from build123d import *

# Parameters (mm, degrees)
SKETCH3_W           = 304.8
SKETCH3_H           = 669.93516
SKETCH3_W_2         = 25.4
SKETCH3_H_2         = 3.175
SKETCH3_W_3         = 3.175
SKETCH3_H_3         = 25.4
BOSS_EXTRUDE1_DEPTH = 3.175
SKETCH6_W           = 107.287119944
SKETCH6_H           = 30.1625
SKETCH6_W_2         = 38.1
SKETCH6_H_2         = 114.3
BOSS_EXTRUDE2_DEPTH = 3.175


with BuildPart() as part:
    # Sketch3 → Boss-Extrude1 (new body)
    with BuildSketch(Plane(origin=(0, 0, 0), x_dir=(1, 0, 0), z_dir=(0, 1, 0))):
        with Locations((48.58004, 334.96758)):
            Rectangle(SKETCH3_W, SKETCH3_H)
        with Locations((25.4, 448.21094)):
            Rectangle(SKETCH3_W_2, SKETCH3_H_2, mode=Mode.SUBTRACT)
        with Locations((175.58004, 448.21094)):
            Rectangle(SKETCH3_W_2, SKETCH3_H_2, mode=Mode.SUBTRACT)
        with Locations((100.49002, 448.21094)):
            Rectangle(SKETCH3_W_2, SKETCH3_H_2, mode=Mode.SUBTRACT)
        with Locations((100.49002, 647.71016)):
            Rectangle(SKETCH3_W_3, SKETCH3_H_3, mode=Mode.SUBTRACT)
        with Locations((100.49002, 475.19844)):
            Rectangle(SKETCH3_W_3, SKETCH3_H_3, mode=Mode.SUBTRACT)
        with Locations((100.49002, 561.4543)):
            Rectangle(SKETCH3_W_3, SKETCH3_H_3, mode=Mode.SUBTRACT)
        with Locations((100.49002, 421.22344)):
            Rectangle(SKETCH3_W_3, SKETCH3_H_3, mode=Mode.SUBTRACT)
        with Locations((100.49002, 334.96758)):
            Rectangle(SKETCH3_W_3, SKETCH3_H_3, mode=Mode.SUBTRACT)
        with Locations((100.49002, 248.71172)):
            Rectangle(SKETCH3_W_3, SKETCH3_H_3, mode=Mode.SUBTRACT)
        with Locations((25.4, 221.72422)):
            Rectangle(SKETCH3_W_2, SKETCH3_H_2, mode=Mode.SUBTRACT)
        with Locations((100.49002, 221.72422)):
            Rectangle(SKETCH3_W_2, SKETCH3_H_2, mode=Mode.SUBTRACT)
        with Locations((175.58004, 221.72422)):
            Rectangle(SKETCH3_W_2, SKETCH3_H_2, mode=Mode.SUBTRACT)
        with Locations((100.49002, 22.225)):
            Rectangle(SKETCH3_W_3, SKETCH3_H_3, mode=Mode.SUBTRACT)
        with Locations((100.49002, 108.48086)):
            Rectangle(SKETCH3_W_3, SKETCH3_H_3, mode=Mode.SUBTRACT)
        with Locations((100.49002, 194.73672)):
            Rectangle(SKETCH3_W_3, SKETCH3_H_3, mode=Mode.SUBTRACT)
        with Locations((-1.59258, 647.71016)):
            Rectangle(SKETCH3_W_3, SKETCH3_H_3, mode=Mode.SUBTRACT)
        with Locations((-1.59258, 475.19844)):
            Rectangle(SKETCH3_W_3, SKETCH3_H_3, mode=Mode.SUBTRACT)
        with Locations((-1.59258, 334.96758)):
            Rectangle(SKETCH3_W_3, SKETCH3_H_3, mode=Mode.SUBTRACT)
        with Locations((-1.59258, 194.73672)):
            Rectangle(SKETCH3_W_3, SKETCH3_H_3, mode=Mode.SUBTRACT)
        with Locations((-1.59258, 22.225)):
            Rectangle(SKETCH3_W_3, SKETCH3_H_3, mode=Mode.SUBTRACT)
    extrude(amount=BOSS_EXTRUDE1_DEPTH)

    # Sketch6 → Boss-Extrude2 (add)
    with BuildSketch(Plane(origin=(0, 3.175, 0), x_dir=(1, 0, 0), z_dir=(0, 1, 0))):
        with Locations((147.336480028, 685.01641)):
            Rectangle(SKETCH6_W, SKETCH6_H)
        with Locations((147.336480028, -15.08125)):
            Rectangle(SKETCH6_W, SKETCH6_H)
        with Locations((-122.86996, 612.78516)):
            Rectangle(SKETCH6_W_2, SKETCH6_H_2)
        with Locations((-122.86996, 57.15)):
            Rectangle(SKETCH6_W_2, SKETCH6_H_2)
    extrude(amount=-BOSS_EXTRUDE2_DEPTH)


solid = part.part
The model under review builds one solid part; all positions refer to its coordinate system, in mm. Give positions to 0.01 mm unless a question says otherwise; leave off trailing zeros. Order: outer loops, then holes, each group sorted by start corner. A loop starts at its lowest first (then second) coordinate and runs counter-clockwise, first axis right, second up. Notation, with made-up numbers: M -18.5,-15.75 L 30.5,-15.75 A18 ccw 30.5,-1.75 Z; hole C -11,74.25 d5. An arc over 180 degrees is marked long. Use one line per item in the form item = value. Start each with the question number.
Item 1: We need section B-B on x = -119. Give the boundary of the cut face in (y, z) (3 decimals).
Item 2: Insertion check: pin 1 Ø1 at (y, z) = (1, -195.5) entering from -X; pin 2 Ø1.6 at (x, y) = (-124, 1) entering from +Z; pin 3 Ø8 at (x, z) = (47.5, -419) entering from -Y. Each pin has a flat end and moves straight along its axis. Give the tip position at first contact, or say it passes through.
Item 3: We need section C-C on y = 0.55. Give the number of separate pieces and of enclosed holes in the cut face, plus the area to 3 significant figures.
Item 4: To check wall thickness, follow line 1 along Z through (x, y) = (97.5, 2.55); line 2 along X through (y, z) = (2.4, -470.5); line 3 along X through (y, z) = (2.2, -651). State the ranges of each line that lie inside material, in increasing order. Write a range as from..to.
Item 5: We need section D-D on x = 78.5. Give the boundary of the cut face in (y, z) (3 decimals).
Item 6: We need section A-A on z = -641.5. Give the boundary of the cut face in (x, y) (3 decimals).
Completed:
q1.outline = M 0,-669.935 L 3.175,-669.935 L 3.175,-555.635 L 0,-555.635 Z; M 0,-114.3 L 3.175,-114.3 L 3.175,0 L 0,0 Z
q2.pin_1 = -103.82
q2.pin_2 = 0
q2.pin_3 = 0
q3.separate_pieces = 1
q3.enclosed_holes = 20
q3.area = 218,000 mm²
q4.line_1 = -700.1..-449.8, -446.62..-223.31, -220.14..30.16
q4.line_2 = -103.82..-3.18, -0.01..98.9, 102.08..200.98
q4.line_3 = -141.92..-3.18, -0.01..98.9, 102.08..200.98
q5.outline = M 0,-669.935 L 3.175,-669.935 L 3.175,0 L 0,0 Z
q6.outline = M -141.92,0 L -3.18,0 L -3.18,3.175 L -141.92,3.175 Z; M -0.005,0 L 98.903,0 L 98.903,3.175 L -0.005,3.175 Z; M 102.078,0 L 200.98,0 L 200.98,3.175 L 102.078,3.175 Z
